Autodesk Inventor part; units mm, degrees
ref_plane "Work Plane1" through (-16.825, 25, 0) normal (0, 0, 1) x (1, 0, 0)
ref_plane "YZ Plane" through (0, 0, 0) normal (1, 0, 0) x (0, 1, 0)
ref_plane "XZ Plane" through (0, 0, 0) normal (0, 1, 0) x (-1, 0, 0)
sketch "Sketch1" plane through (0, 0, 0) normal (0, 1, 0) x (-1, 0, 0)
  line L0 (-12.5, -44) -> (12.5, -44)
  line L1 (12.5, -44) -> (12.5, 44)
  line L2 (12.5, 44) -> (-12.5, 44)
  line L3 (-12.5, 44) -> (-12.5, -44)
  line L4 (-12.5, -44) -> (12.5, 44) construction
  line L5 (12.5, -44) -> (-12.5, 44) construction
  point P0 (0, 0)
  dimension "d0" = 88
  dimension "d1" = 25
extrude "Extrusion1" add sketch "Sketch1" along normal blind 9.525
sketch "Sketch2" plane through (0, 9.525, 0) normal (0, 1, 0) x (1, 0, 0)
  line L0 (20, -34.475) -> (-20, -34.475)
  line L1 (-20, -34.475) -> (-20, -44)
  line L2 (-20, -44) -> (20, -44)
  line L3 (20, -44) -> (20, -34.475)
  line L4 (20, -34.475) -> (-20, -44) construction
  line L5 (-20, -34.475) -> (20, -44) construction
  line L6 (-12.5, -44) -> (12.5, -44)
  point P0 (0, 0)
  point P1 (0, -39.2375)
  dimension "d4" = 40
  dimension "d5" = 9.525
extrude "Extrusion2" add sketch "Sketch2" along normal blind 15.475
fillet "Fillet1" radius 3.175 6 edges at (-12.5, 9.525, 39.2375) (-20, 9.525, 39.2375) (-20, 25, 39.2375) (20, 9.525, 39.2375) (20, 25, 39.2375) (12.5, 9.525, 39.2375)
ref_plane "Work Plane1" through (-16.825, 25, 0) normal (0, 0, 1) x (1, 0, 0)
mirror "Mirror1" about plane through (-16.825, 25, 0) normal (0, 0, 1) of "Extrusion2", "Fillet1"
sketch "Sketch3" plane through (16.825, 25, -44) normal (0, 0, -1) x (-1, 0, 0)
  line L0 (29.325, -25) -> (29.325, -18.65)
  arc A0 (32.5, -15.475) -> (29.325, -18.65) centre (32.5, -18.65) ccw
  line L1 (33.65, -15.475) -> (32.5, -15.475)
  arc A1 (33.65, -15.475) -> (36.825, -12.3) centre (33.65, -12.3) ccw
  line L2 (36.825, -12.3) -> (36.825, -3.175)
  arc A2 (36.825, -3.175) -> (33.65, 0) centre (33.65, -3.175) ccw
  line L3 (33.65, 0) -> (0, 0)
  arc A3 (0, 0) -> (-3.175, -3.175) centre (0, -3.175) ccw
  line L4 (-3.175, -12.3) -> (-3.175, -3.175)
  arc A4 (-3.175, -12.3) -> (0, -15.475) centre (0, -12.3) ccw
  line L5 (1.15, -15.475) -> (0, -15.475)
  arc A5 (4.325, -18.65) -> (1.15, -15.475) centre (1.15, -18.65) ccw
  line L6 (4.325, -25) -> (4.325, -18.65)
  circle A6 centre (26.825, -10) radius 2.6
  circle A7 centre (6.825, -10) radius 2.6
  line L7 (4.325, -25) -> (29.325, -25)
  point P0 (16.825, -25)
  dimension "d10" = 5.2
  dimension "d11" = 10
  dimension "d12" = 10
  dimension "d13" = 10
extrude "Extrusion3" cut sketch "Sketch3" against normal through all contours A6 | A7
sketch "Sketch4" plane through (0, 0, 0) normal (0, -1, 0) x (1, 0, 0)
  line L0 (-6.5, -23) -> (6.5, -23) construction
  line L1 (6.5, -23) -> (6.5, 23) construction
  line L2 (6.5, 23) -> (-6.5, 23) construction
  line L3 (-6.5, 23) -> (-6.5, -23) construction
  line L4 (-6.5, -23) -> (6.5, 23) construction
  line L5 (6.5, -23) -> (-6.5, 23) construction
  circle A0 centre (6.5, 23) radius 2.6
  circle A1 centre (6.5, -23) radius 2.6
  circle A2 centre (-6.5, -23) radius 2.6
  circle A3 centre (-6.5, 23) radius 2.6
  point P0 (0, 0)
  dimension "d16" = 5.2
  dimension "d17" = 46
  dimension "d18" = 13
extrude "Extrusion4" cut sketch "Sketch4" against normal through all
sketch "Sketch5" plane through (16.825, 25, -44) normal (0, 0, -1) x (-1, 0, 0)
  circle A0 centre (6.825, -10) radius 2.6
  circle A1 centre (26.825, -10) radius 2.6
  line L0 (5.3878, -7.8333) -> (6.825, -6.88)
  line L1 (6.825, -6.88) -> (8.2622, -7.8333)
  line L2 (25.3878, -7.8333) -> (26.825, -6.88)
  line L3 (26.825, -6.88) -> (28.2622, -7.8333)
  point P0 (16.825, -25)
  point P1 (6.825, -7.4)
  point P2 (26.825, -7.4)
  dimension "d21" = 0.52
  dimension "d22" = 5.2
  dimension "d23" = 0.52
extrude "Extrusion5" cut sketch "Sketch5" against normal through all contours A0 L0 L1 | A1 L2 L3
sketch "Sketch6" plane through (0, 9.525, 0) normal (0, 1, 0) x (1, 0, 0)
  circle A0 centre (-6.5, 23) radius 2.6
  circle A1 centre (6.5, 23) radius 2.6
  circle A2 centre (-6.5, -23) radius 2.6
  circle A3 centre (6.5, -23) radius 2.6
  circle A4 centre (-6.5, 23) radius 5
  circle A5 centre (6.5, 23) radius 5
  circle A6 centre (-6.5, -23) radius 5
  circle A7 centre (6.5, -23) radius 5
  point P0 (0, 0)
  dimension "d26" = 10
extrude "Extrusion6" add sketch "Sketch6" against normal up to surface (9.525 mm away)
chamfer "Chamfer1" distance 3.175 angle 45 2 edges at (0, 0, -44) (0, 0, 44)
sketch "Sketch7" plane through (-16.825, 25, 44) normal (0, 0, 1) x (1, 0, 0)
  line L0 (29.325, -21.825) -> (4.325, -21.825)
  line L1 (29.325, -21.825) -> (29.325, -18.65)
  arc A0 (32.5, -15.475) -> (29.325, -18.65) centre (32.5, -18.65) ccw
  line L2 (32.5, -15.475) -> (33.65, -15.475)
  arc A1 (33.65, -15.475) -> (36.825, -12.3) centre (33.65, -12.3) ccw
  line L3 (36.825, -12.3) -> (36.825, -3.175)
  arc A2 (36.825, -3.175) -> (33.65, 0) centre (33.65, -3.175) ccw
  line L4 (0, 0) -> (33.65, 0)
  arc A3 (0, 0) -> (-3.175, -3.175) centre (0, -3.175) ccw
  line L5 (-3.175, -12.3) -> (-3.175, -3.175)
  arc A4 (-3.175, -12.3) -> (0, -15.475) centre (0, -12.3) ccw
  line L6 (0, -15.475) -> (1.15, -15.475)
  arc A5 (4.325, -18.65) -> (1.15, -15.475) centre (1.15, -18.65) ccw
  line L7 (4.325, -21.825) -> (4.325, -18.65)
  line L8 (5.3878, -7.8333) -> (6.825, -6.88)
  line L9 (6.825, -6.88) -> (8.2622, -7.8333)
  arc A6 (5.3878, -7.8333) -> (8.2622, -7.8333) centre (6.825, -10) ccw
  line L10 (25.3878, -7.8333) -> (26.825, -6.88)
  line L11 (26.825, -6.88) -> (28.2622, -7.8333)
  arc A7 (25.3878, -7.8333) -> (28.2622, -7.8333) centre (26.825, -10) ccw
  line L12 (-3.175, 0) -> (36.825, 0)
  line L13 (36.825, 0) -> (36.825, -15.475)
  line L14 (36.825, -15.475) -> (-3.175, -15.475)
  line L15 (-3.175, -15.475) -> (-3.175, 0)
  line L16 (0, 0) -> (33.65, 0)
  line L17 (36.825, -12.3) -> (36.825, -3.175)
  line L18 (32.5, -15.475) -> (33.65, -15.475)
  line L19 (-3.175, -12.3) -> (-3.175, -3.175)
  line L20 (29.325, -18.65) -> (29.325, -15.475)
  line L21 (4.325, -18.65) -> (4.325, -15.475)
  point P0 (16.825, -25)
  point P1 (0, -15.475)
extrude "Extrusion7" add sketch "Sketch7" against normal up to surface (9.525 mm away) contours A1 L13 L14 | L14 L15 A4 | A2 L12 L13 | L15 L12 A3
extrude "Extrusion8" cut sketch "Sketch7" against normal through all contours L20 L14 A0 | A5 L14 L21
sketch "Sketch8" plane through (20, 25, 34.475) normal (0, 0, -1) x (-1, 0, 0)
  line L0 (7.5, -15.475) -> (7.5, -18.65)
  arc A0 (10.675, -15.475) -> (7.5, -18.65) centre (10.675, -18.65) ccw
  line L1 (29.325, -15.475) -> (10.675, -15.475)
  arc A1 (32.5, -18.65) -> (29.325, -15.475) centre (29.325, -18.65) ccw
  line L2 (32.5, -18.65) -> (32.5, -15.475)
  line L3 (40, -15.475) -> (32.5, -15.475)
  line L4 (40, 0) -> (40, -15.475)
  line L5 (0, 0) -> (40, 0)
  line L6 (0, -15.475) -> (0, 0)
  line L7 (0, -15.475) -> (7.5, -15.475)
  line L8 (8.5628, -7.8333) -> (10, -6.88)
  line L9 (10, -6.88) -> (11.4372, -7.8333)
  arc A2 (8.5628, -7.8333) -> (11.4372, -7.8333) centre (10, -10) ccw
  line L10 (28.5628, -7.8333) -> (30, -6.88)
  line L11 (30, -6.88) -> (31.4372, -7.8333)
  arc A3 (28.5628, -7.8333) -> (31.4372, -7.8333) centre (30, -10) ccw
  line L12 (7.5, -15.475) -> (32.5, -15.475)
  point P0 (20, -25)
  point P1 (10.675, -15.475)
extrude "Extrusion9" add sketch "Sketch8" along normal up to surface (68.95 mm away) contours L12 A0 L0 | L12 L2 A1
mirror "Mirror2" about plane through (-16.825, 25, 0) normal (0, 0, 1) of "Extrusion2"
chamfer "Chamfer2" distance 1.5875 angle 45 14 edges at (20, 25, 39.2375) (20, 9.525, 39.2375) (-20, 25, 39.2375) (-20, 9.525, 39.2375) (-12.5, 9.525, 39.2375) (-12.5, 9.525, -39.2375) (-20, 9.525, -39.2375) (-20, 25, -39.2375) (12.5, 9.525, -39.2375) (12.5, 9.525, 39.2375) (20, 25, -39.2375) (20, 9.525, -39.2375) (-12.5, 9.525, 0) (12.5, 9.525, 0)
equation "\"d12\" = d11"
equation "\"d13\" = d12"
properties part number "CNC-023-YAxisBallScrewStabilizerMount" material "ABS Plastic"
Here's how the part is built. I have some questions about the finished solid (model axes, mm). A direction names the side the tool comes from. Coordinates: 2 decimals unless noted, no trailing zeros. Order: outer loops, then holes, each group sorted by start corner. A loop starts at its lowest first (then second) coordinate and runs counter-clockwise, first axis right, second up.
Item 1: If we section it at D-D, the plane x = -6.5: List the corners of the cut face in (y, z) for me (3 decimals).
Response values:
outline: (0, -40.825) - (3.175, -44) - (25, -44) - (25, -34.475) - (9.525, -34.475) - (9.525, -25.6) - (0, -25.6) - close; (0, -20.4) - (9.525, -20.4) - (9.525, 20.4) - (0, 20.4) - close; (0, 25.6) - (9.525, 25.6) - (9.525, 34.475) - (25, 34.475) - (25, 44) - (3.175, 44) - (0, 40.825) - close
Item 2: I need wall thicknesses on probe 1 along X at (y, z) = (15, 40); probe 2 along Z at (x, y) = (6.5, 6); probe 3 along Z at (x, y) = (-11, 21) (3 decimals). Which ranges of each line are inside material? Lowest first, please.
Response values:
probe 1: x = -20 to -12.6, -7.4 to 7.4, 12.6 to 20
probe 2: z = -44 to -25.6, -20.4 to 20.4, 25.6 to 44
probe 3: z = -44 to -34.475, 34.475 to 44
Item 3: I'm going to push flat-ended pins straight in: pin 1 Ø2 at (x, z) = (16, -40.5) entering from -Y (3 decimals); pin 2 Ø12 at (y, z) = (15, -24) entering from +X; pin 3 Ø4.5 at (x, z) = (6.5, 23) entering from -Y; pin 4 Ø12 at (x, z) = (-0.5, 8) entering from +Y (3 decimals). Where does each tip first touch, or does it pass through?
Response values:
pin 1: stops at y = 9.525
pin 2: stops at x = 11.44
pin 3: passes through
pin 4: stops at y = 9.525
Item 4: If we section it at B-B, the plane y = 15: List the corners of the cut face in (x, z) for me (3 decimals).
Response values:
outline: (-20, -44) - (20, -44) - (20, -34.475) - (-20, -34.475) - close; (-20, 34.475) - (-12.6, 34.475) - (-12.6, 44) - (-20, 44) - close; (-7.4, 34.475) - (7.4, 34.475) - (7.4, 44) - (-7.4, 44) - close; (12.6, 34.475) - (20, 34.475) - (20, 44) - (12.6, 44) - close
Item 5: Thinking about a two-plate mould opening in Z: for faces 5 (the face through (0, 14, -44)), 6 (the face through (16, 9.525, -39)), 7 (the face through (-11.72, 8.72, -0.48)), which applies, pulls with the +Z half, pulls with the -Z half, needs draft (parallel to the pull), parting line crosses it, or undercut?
Response values:
face 5: pulls with the -Z half
face 6: needs draft
face 7: undercut
Item 6: Which directions (+Z, -Z, +X, -X, +Y, -Y) give clear straight access to the entire face, cutting with the end or side of a thin tool? Please do faces 1 (the face through (-9.9, 12.4, 39.2)), 2 (the face through (-16, 9.525, -39)), 3 (the face through (0, 9.525, 0)), 4 (the face through (-19.217, 24.195, 39.171)).
Response values:
face 1: +Z
face 2: +Z, -Z, -X, -Y
face 3: +X, -X, +Y
face 4: +Z, -Z, -X, +Y
Item 7: If we section it at A-A, the plane z = -23: List the corners of the cut face in (x, y) for me (1 decimal).
Response values:
outline: (-12.5, 0) - (-9.1, 0) - (-9.1, 9.5) - (-10.9, 9.5) - (-12.5, 7.9) - close; (-3.9, 0) - (3.9, 0) - (3.9, 9.5) - (-3.9, 9.5) - close; (9.1, 0) - (12.5, 0) - (12.5, 7.9) - (10.9, 9.5) - (9.1, 9.5) - close
Item 8: If we section it at C-C, the plane y = 20.25: List the corners of the cut face in (x, z) for me (3 decimals), then the cut area to 3 significant figures.
Response values:
outline: (-20, -44) - (20, -44) - (20, -34.475) - (-20, -34.475) - close; (-20, 34.475) - (20, 34.475) - (20, 44) - (-20, 44) - close
area: 762 mm2
